Here's how the part is built. I have some questions about the finished solid (model axes, mm). A direction names the side the tool comes from. Coordinates: 2 decimals unless noted, no trailing zeros. Write each loop counter-clockwise with the first axis right and the second up, starting at its lowest first coordinate (ties: lowest second). Pieces come first, ordered by that corner, then holes.
Item 1: For faces 1 (the face through (15, 1, -6.21)), 2 (the face through (-16.52, 4, 48)), which set-ups out of +Z, -Z, +X, -X, +Y, -Y let a thin tool reach every point of the face, with its end or its side?
Item 2: I want a section at A-A (z = 42). Please give me the cut outline in (x, y), and give its area (3 significant figures).
Item 3: If we mould it in two halves opening along Z, with no side actions, what happens to faces 3 (the face through (-47.14, -7, 47)), 4 (the face through (-53, 3, 54)), 5 (the face through (25.84, 3, -26))? For each: pulls with the +Z half, pulls with the -Z half, needs draft (parallel to the pull), parting line crosses it, or undercut.
Item 4: I'm going to push flat-ended pins straight in: P1, Ø6, axis at x = 43.5, y = -6, coming from the +Z side; P2, Ø3.5, axis at x = 20.54, z = -50.81, coming from the -Y side; P3, Ø5.5, axis at x = -35, z = 35, coming from the -Y side; P4, Ø2, axis at x = -15, y = -4, coming from the +Z side. Where does each tip first touch, or does it pass through?
Item 5: Please list where these lines run through material, in increasing order: line 1 (X direction, y = 3.8, z = -10.55); line 2 (X direction, y = 2.7, z = 10.55); line 3 (X direction, y = 4.25, z = 16).
Item 6: I want a section at C-C (z = -44). Please give me the cut outline in (x, y).
Item 7: I want a section at B-B (z = 20.55). Please give me the cut outline in (x, y), and give its area (3 significant figures).
from build123d import *

# Parameters (mm, degrees)
SKETCH_1_W                 = 110
SKETCH_1_H                 = 110
EXTRUDE_1_DEPTH            = 5
SKETCH_2_R                 = 2.25
SKETCH_2_W                 = 40.6
SKETCH_2_H                 = 20.6
SKETCH_2_W_2               = 20.6
SKETCH_2_H_2               = 40.6
CUT_EXTRUDE_1_DEPTH        = 5
SKETCH_4_R                 = 1.65
CUT_EXTRUDE_2_DEPTH        = 5
CUT_EXTRUDE_3_DEPTH        = 1
PATTERN_START              = -16.519760508
PATTERN_CIRCULAR_3_DEPTH   = 1.959837541
PATTERN_START_2            = 14.653884875
PATTERN_CIRCULAR_3_2_DEPTH = 1.922796081
PATTERN_START_3            = 16.576680956
PATTERN_CIRCULAR_3_3_DEPTH = 0.077203919
PATTERN_START_4            = 14.576680956
PATTERN_CIRCULAR_3_4_DEPTH = 0.077203919
PATTERN_START_5            = -14.559922967
PATTERN_CIRCULAR_3_5_DEPTH = 0.040162459
PATTERN_START_6            = -16.559922967
PATTERN_CIRCULAR_3_6_DEPTH = 0.040162459
PATTERN_START_7            = 14.623645383
PATTERN_CIRCULAR_3_7_DEPTH = 1.96295854
PATTERN_START_8            = 16.586603923
PATTERN_CIRCULAR_3_8_DEPTH = 0.03704146
PATTERN_START_9            = 14.586603923
PATTERN_CIRCULAR_3_9_DEPTH = 0.03704146
SKETCH_9_W                 = 110
SKETCH_9_H                 = 5
EXTRUDE_4_DEPTH            = 20
EXTRUDE_5_DEPTH            = 20
EXTRUDE_6_DEPTH            = 15
CUT_EXTRUDE_4_DEPTH        = 2
FILLET_1_R                 = 2
FILLET_2_R                 = 2
FILLET_3_R                 = 2
SKETCH_13_R                = 2.5
CUT_EXTRUDE_5_DEPTH        = 1
SKETCH_14_R                = 2.5
CUT_EXTRUDE_6_DEPTH        = 1
SKETCH_15_W                = 110
SKETCH_15_H                = 5
CUT_EXTRUDE_7_DEPTH        = 4
FILLET_4_R                 = 5
SKETCH_17_W                = 2
SKETCH_17_H                = 3.5
CUT_EXTRUDE_10_DEPTH       = 4
SKETCH_18_W                = 2
SKETCH_18_H                = 3.5
CUT_EXTRUDE_11_DEPTH       = 4
SKETCH_19_W                = 2
SKETCH_19_H                = 3.5
CUT_EXTRUDE_12_DEPTH       = 4


# Read off the part's stored shape, not the designer's step: 阵列(圆周)3
with BuildPart() as part:
    # 草图1 → 凸台-拉伸1 (new body)
    with BuildSketch(Plane(origin=(0, 0, 0), x_dir=(1, 0, 0), z_dir=(0, 1, 0))):
        Rectangle(SKETCH_1_W, SKETCH_1_H)
    extrude(amount=EXTRUDE_1_DEPTH)

    # 草图2 → 切除-拉伸1 (cut)
    with BuildSketch(Plane(origin=(0, 5, 0), x_dir=(1, 0, 0), z_dir=(0, 1, 0))):
        with Locations(Location((2.2, -10.55, 0), (0, 0, 270))):
            Circle(SKETCH_2_R)
        with Locations(Location((2.2, -20.55, 0), (0, 0, 90))):
            Circle(SKETCH_2_R)
        with Locations(Location((50.8, -20.55, 0), (0, 0, 270))):
            Circle(SKETCH_2_R)
        with Locations(Location((50.8, -10.55, 0), (0, 0, 90))):
            Circle(SKETCH_2_R)
        with Locations(Location((-10.56, -50.81, 0), (0, 0, 90))):
            Circle(SKETCH_2_R)
        with Locations(Location((-20.56, -50.81, 0), (0, 0, 270))):
            Circle(SKETCH_2_R)
        with Locations(Location((-20.56, -2.21, 0), (0, 0, 90))):
            Circle(SKETCH_2_R)
        with Locations(Location((-10.56, -2.21, 0), (0, 0, 270))):
            Circle(SKETCH_2_R)
        with Locations(Location((-50.82, 10.55, 0), (0, 0, 90))):
            Circle(SKETCH_2_R)
        with Locations(Location((-50.82, 20.55, 0), (0, 0, 270))):
            Circle(SKETCH_2_R)
        with Locations(Location((-2.22, 20.55, 0), (0, 0, 90))):
            Circle(SKETCH_2_R)
        with Locations(Location((-2.22, 10.55, 0), (0, 0, 270))):
            Circle(SKETCH_2_R)
        with Locations(Location((10.54, 50.81, 0), (0, 0, 90))):
            Circle(SKETCH_2_R)
        with Locations(Location((20.54, 50.81, 0), (0, 0, 270))):
            Circle(SKETCH_2_R)
        with Locations(Location((20.54, 2.21, 0), (0, 0, 90))):
            Circle(SKETCH_2_R)
        with Locations(Location((10.54, 2.21, 0), (0, 0, 270))):
            Circle(SKETCH_2_R)
        with Locations((-26.52, 15.55)):
            Rectangle(SKETCH_2_W, SKETCH_2_H)
        with Locations((-15.56, -26.51)):
            Rectangle(SKETCH_2_W_2, SKETCH_2_H_2)
        with Locations((26.5, -15.55)):
            Rectangle(SKETCH_2_W, SKETCH_2_H)
        with Locations((15.54, 26.51)):
            Rectangle(SKETCH_2_W_2, SKETCH_2_H_2)
    extrude(amount=-CUT_EXTRUDE_1_DEPTH, mode=Mode.SUBTRACT)

    # 草图4 → 切除-拉伸2 (cut)
    with BuildSketch(Plane(origin=(0, 5, 0), x_dir=(1, 0, 0), z_dir=(0, 1, 0))):
        with Locations(Location((-35, 35, 0), (0, 0, 270))):
            Circle(SKETCH_4_R)
        with Locations(Location((35, 35, 0), (0, 0, 270))):
            Circle(SKETCH_4_R)
        with Locations(Location((35, -35, 0), (0, 0, 270))):
            Circle(SKETCH_4_R)
        with Locations(Location((-35, -35, 0), (0, 0, 270))):
            Circle(SKETCH_4_R)
    extrude(amount=-CUT_EXTRUDE_2_DEPTH, mode=Mode.SUBTRACT)

    # 草图6 → 切除-拉伸3 (cut, symmetric)
    with BuildSketch(Plane.XY.offset(-15.55)):
        Polygon((-46.82, 5), (-51.82, 5), (-46.82, 1.5), align=None)
    cut_extrude_3 = extrude(amount=CUT_EXTRUDE_3_DEPTH, both=True, mode=Mode.SUBTRACT)

    # 镜向1: 切除-拉伸3 across plane
    add(cut_extrude_3.mirror(Plane(origin=(-26.52, 0, 0), x_dir=(0, 0, 1), z_dir=(1, 0, 0))), mode=Mode.SUBTRACT)

    # 阵列(圆周)3 outline → 阵列(圆周)3 (cut)
    with BuildSketch(Plane.YZ.offset(PATTERN_START)):
        Polygon((1.5, 46.923884875), (5, 46.923884875), (5, 51.923884875), align=None)
        Polygon((1.525676669, 6.21), (5, 1.246680956), (5, 6.21), align=None)
    extrude(amount=PATTERN_CIRCULAR_3_DEPTH, mode=Mode.SUBTRACT)

    # Pattern Circular 3 2 outline → Pattern Circular 3 2 (cut)
    with BuildSketch(Plane.YZ.offset(PATTERN_START_2)):
        Polygon((5, -51.850239492), (5, -46.850239492), (1.5, -46.850239492), align=None)
        Polygon((1.500053923, -6.21), (5, -6.21), (5, -1.210077033), align=None)
    extrude(amount=PATTERN_CIRCULAR_3_2_DEPTH, mode=Mode.SUBTRACT)

    # Pattern Circular 3 3 outline → Pattern Circular 3 3 (cut)
    with BuildSketch(Plane.YZ.offset(PATTERN_START_3)):
        Polygon((5, -51.850239492), (5, -46.850239492), (1.5, -46.850239492), align=None)
    extrude(amount=PATTERN_CIRCULAR_3_3_DEPTH, mode=Mode.SUBTRACT)

    # Pattern Circular 3 4 outline → Pattern Circular 3 4 (cut)
    with BuildSketch(Plane.YZ.offset(PATTERN_START_4)):
        Polygon((1.500053923, -6.21), (5, -6.21), (5, -1.210077033), align=None)
    extrude(amount=PATTERN_CIRCULAR_3_4_DEPTH, mode=Mode.SUBTRACT)

    # Pattern Circular 3 5 outline → Pattern Circular 3 5 (cut)
    with BuildSketch(Plane.YZ.offset(PATTERN_START_5)):
        Polygon((1.5, 46.923884875), (5, 46.923884875), (5, 51.923884875), align=None)
    extrude(amount=PATTERN_CIRCULAR_3_5_DEPTH, mode=Mode.SUBTRACT)

    # Pattern Circular 3 6 outline → Pattern Circular 3 6 (cut)
    with BuildSketch(Plane.YZ.offset(PATTERN_START_6)):
        Polygon((1.525676669, 6.21), (5, 1.246680956), (5, 6.21), align=None)
    extrude(amount=PATTERN_CIRCULAR_3_6_DEPTH, mode=Mode.SUBTRACT)

    # Pattern Circular 3 7 outline → Pattern Circular 3 7 (cut)
    with BuildSketch(Plane.XY.offset(PATTERN_START_7)):
        Polygon((51.954124367, 5), (46.954124367, 5), (46.954124367, 1.5), align=None)
        Polygon((6.2, 1.525730592), (6.2, 5), (1.236757989, 5), align=None)
    extrude(amount=PATTERN_CIRCULAR_3_7_DEPTH, mode=Mode.SUBTRACT)

    # Pattern Circular 3 8 outline → Pattern Circular 3 8 (cut)
    with BuildSketch(Plane.XY.offset(PATTERN_START_8)):
        Polygon((51.954124367, 5), (46.954124367, 5), (46.954124367, 1.5), align=None)
    extrude(amount=PATTERN_CIRCULAR_3_8_DEPTH, mode=Mode.SUBTRACT)

    # Pattern Circular 3 9 outline → Pattern Circular 3 9 (cut)
    with BuildSketch(Plane.XY.offset(PATTERN_START_9)):
        Polygon((6.2, 1.525730592), (6.2, 5), (1.236757989, 5), align=None)
    extrude(amount=PATTERN_CIRCULAR_3_9_DEPTH, mode=Mode.SUBTRACT)

    # 草图9 → 凸台-拉伸4 (add)
    with BuildSketch(Plane(origin=(0, 0, -55), x_dir=(-1, 0, 0), z_dir=(0, 0, -1))):
        with Locations((0, 2.5)):
            Rectangle(SKETCH_9_W, SKETCH_9_H)
    extrude(amount=EXTRUDE_4_DEPTH)

    # 草图10 → 凸台-拉伸5 (add)
    with BuildSketch(Plane(origin=(0, 5, 0), x_dir=(1, 0, 0), z_dir=(0, 1, 0))):
        Polygon((26.679814029, 60.6), (12.667174987, 65.571224494), (31.679814029, 65.571224494), (31.679814029, 56.6), (-31.679814029, 56.6), (-31.679814029, 65.571224494), (-12.667174987, 65.571224494), (-26.679814029, 60.6), align=None)
    extrude(amount=-EXTRUDE_5_DEPTH)

    # 草图11 → 凸台-拉伸6 (add)
    with BuildSketch(Plane.XZ):
        Polygon((47.14, 44.39), (47.14, 49.39), (51.14, 49.39), (51.14, 40.39), (25.757217781, 40.39), (25.757217781, 49.39), (39.507217781, 49.39), (30.757217781, 44.39), align=None)
    extrude_6 = extrude(amount=EXTRUDE_6_DEPTH)

    # 镜向2: 凸台-拉伸6 across plane
    add(extrude_6.mirror(Plane(origin=(0, 0, 0), x_dir=(0, 0, 1), z_dir=(1, 0, 0))))

    # 草图12 → 切除-拉伸4 (cut)
    with BuildSketch(Plane(origin=(-25.757217781, 0, 0), x_dir=(0, 0, -1), z_dir=(1, 0, 0))):
        Polygon((-46.81, 0), (-49.39, 0), (-49.39, -15), (-40.39, -15), (-40.39, 0), align=None)
    extrude(amount=-CUT_EXTRUDE_4_DEPTH, mode=Mode.SUBTRACT)

    # 圆角1
    fillet_1_edges = [part.edges().sort_by_distance(p)[0] for p in [
        (-51.14, 0, 44.89),
        (-49.14, 0, 49.39),
        (-33.632217781, 0, 49.39),
        (-39.448608891, 0, 40.39),
    ]]
    fillet(fillet_1_edges, radius=FILLET_1_R)

    # 圆角2
    fillet_2_edges = [part.edges().sort_by_distance(p)[0] for p in [
        (32.632217781, 0, 49.39),
        (25.757217781, 0, 44.89),
        (38.448608891, 0, 40.39),
        (51.14, 0, 44.89),
        (49.14, 0, 49.39),
    ]]
    fillet(fillet_2_edges, radius=FILLET_2_R)

    # 圆角3
    fillet_3_edges = [part.edges().sort_by_distance(p)[0] for p in [
        (-22.173494508, 0, -65.571224494),
        (-31.679814029, 0, -61.085612247),
        (0, 0, -56.6),
        (31.679814029, 0, -61.085612247),
        (22.173494508, 0, -65.571224494),
    ]]
    fillet(fillet_3_edges, radius=FILLET_3_R)

    # 草图13 → 切除-拉伸5 (cut)
    with BuildSketch(Plane(origin=(0, 0, -60.6), x_dir=(-1, 0, 0), z_dir=(0, 0, -1))):
        with Locations((0, -8)):
            Circle(SKETCH_13_R)
    extrude(amount=-CUT_EXTRUDE_5_DEPTH, mode=Mode.SUBTRACT)

    # 草图14 → 切除-拉伸6 (cut)
    with BuildSketch(Plane.XY.offset(44.39)):
        with Locations((43.66, -8)):
            Circle(SKETCH_14_R)
    cut_extrude_6 = extrude(amount=-CUT_EXTRUDE_6_DEPTH, mode=Mode.SUBTRACT)

    # 镜向4: 切除-拉伸6 across plane
    add(cut_extrude_6.mirror(Plane(origin=(0, 0, 0), x_dir=(0, 0, 1), z_dir=(1, 0, 0))), mode=Mode.SUBTRACT)

    # 草图15 → 切除-拉伸7 (cut)
    with BuildSketch(Plane(origin=(0, 0, -75), x_dir=(-1, 0, 0), z_dir=(0, 0, -1))):
        with Locations((0, 2.5)):
            Rectangle(SKETCH_15_W, SKETCH_15_H)
    extrude(amount=-CUT_EXTRUDE_7_DEPTH, mode=Mode.SUBTRACT)

    # 圆角4
    fillet_4_edges = [part.edges().sort_by_distance(p)[0] for p in [
        (-55, 2.5, -71),
        (55, 2.5, -71),
        (55, 2.5, 55),
        (-55, 2.5, 55),
    ]]
    fillet(fillet_4_edges, radius=FILLET_4_R)

    # 草图17 → 切除-拉伸10 (cut)
    with BuildSketch(Plane(origin=(0, 0, -46.850239492), x_dir=(-1, 0, 0), z_dir=(0, 0, -1))):
        with Locations((-15.653884875, 3.25)):
            Rectangle(SKETCH_17_W, SKETCH_17_H)
    extrude(amount=-CUT_EXTRUDE_10_DEPTH, mode=Mode.SUBTRACT)

    # 草图18 → 切除-拉伸11 (cut)
    with BuildSketch(Plane.XY.offset(46.923884875)):
        with Locations((-15.519760508, 3.25)):
            Rectangle(SKETCH_18_W, SKETCH_18_H)
    extrude(amount=-CUT_EXTRUDE_11_DEPTH, mode=Mode.SUBTRACT)

    # 草图19 → 切除-拉伸12 (cut)
    with BuildSketch(Plane(origin=(46.954124367, 0, 0), x_dir=(0, 0, -1), z_dir=(1, 0, 0))):
        with Locations((-15.623645383, 3.25)):
            Rectangle(SKETCH_19_W, SKETCH_19_H)
    extrude(amount=-CUT_EXTRUDE_12_DEPTH, mode=Mode.SUBTRACT)


solid = part.part
Answer:
1. face 1: +Y, -Y
1. face 2: +Y
2. outline: (-55, 0) - (-53.14, 0) arc R2 cw to (-51.14, -2) - (-51.14, -15) - (-27.76, -15) - (-27.76, 0) - (-25.86, 0) - (-25.86, 5) - (-55, 5) - close; (-5.26, 0) - (23.76, 0) arc R2 cw to (25.76, -2) - (25.76, -15) - (51.14, -15) - (51.14, -2) arc R2 cw to (53.14, 0) - (55, 0) - (55, 5) - (-5.26, 5) - close
2. area: 1,180 mm2
3. face 3: needs draft
3. face 4: pulls with the +Z half
3. face 5: undercut
4. P1: stops at z = 44.39
4. P2: passes through
4. P3: stops at y = 0
4. P4: stops at z = -56.6
5. line 1: x = -55 to -53.07, -48.57 to -46.82, -6.22 to -4.47, 0.03 to 5.24, 25.84 to 55
5. line 2: x = -55 to -25.86, -5.26 to -0.05, 4.45 to 6.2, 46.8 to 48.55, 53.05 to 55
5. line 3: x = -55 to -25.86, -5.26 to 2.31, 50.88 to 55
6. outline: (-55, 0) - (5.24, 0) - (5.24, 5) - (-55, 5) - close; (25.84, 0) - (55, 0) - (55, 5) - (25.84, 5) - close
7. outline: (-55, 0) - (-25.86, 0) - (-25.86, 5) - (-55, 5) - close; (-5.26, 0) - (-0.05, 0) - (-0.05, 5) - (-5.26, 5) - close; (4.45, 0) - (6.2, 0) - (6.2, 5) - (4.45, 5) - close; (46.8, 0) - (48.55, 0) - (48.55, 5) - (46.8, 5) - close; (53.05, 0) - (55, 0) - (55, 5) - (53.05, 5) - close
7. area: 199 mm2
